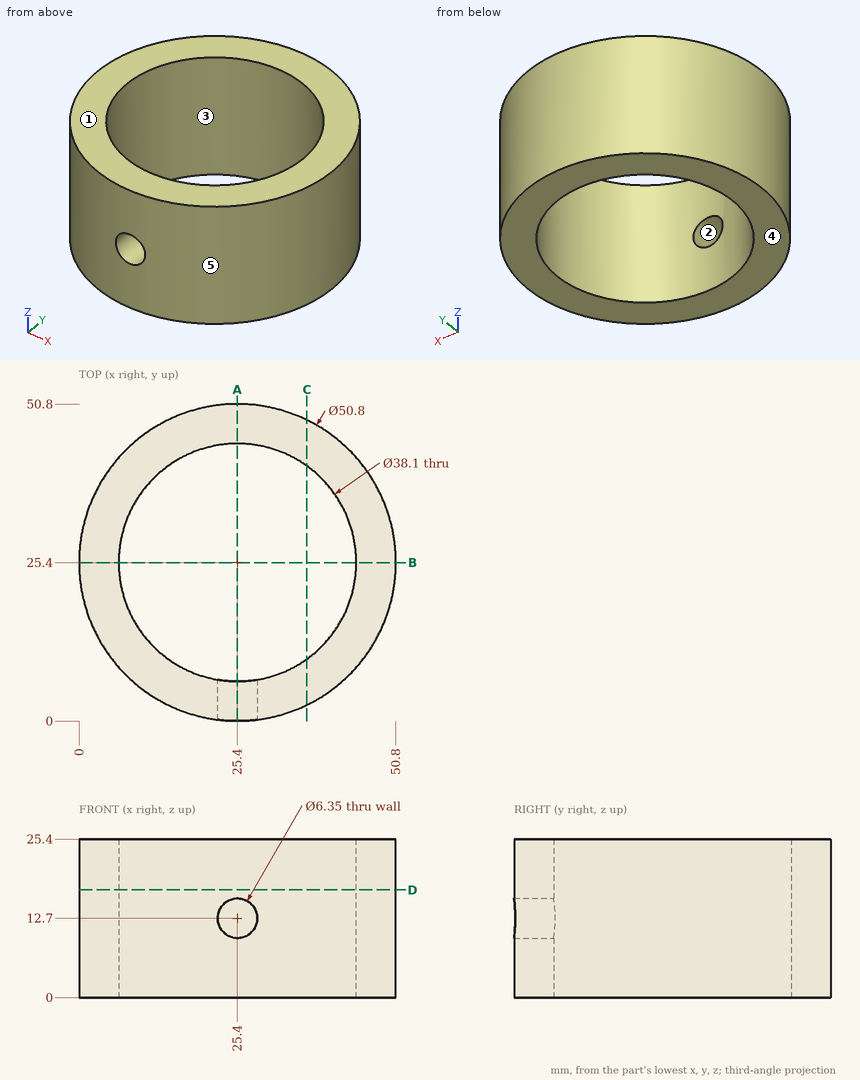
The drawing under review shows one solid part. Ordinate dimensions are in mm from its lowest x, y, z. A direction names the side the tool comes from. Round coordinates to 2 decimals unless told otherwise and drop trailing zeros. Loops run counter-clockwise (first coordinate to the right, second up) from the corner with the lowest first, then second, coordinate; pieces in that order, holes last. Notation, with made-up numbers: (-1.5, 9.5) -> (39.5, 9.5) arc R34 ccw to (39.5, 40.5) -> close; hole circle Ø10 at (-2, 2.25). An arc over 180 degrees is marked (long way). One line per question, with ' | ' between items. Start each with the question number.
Item 1: Add section A-A, the plane x = 25.4. Write out the cut boundary in (y, z) (3 decimals).
Item 2: Draft analysis for pull direction X (two halves, no side actions). For the marked faces 3, 4 and 5, state which applies: +X half, -X half, draft (parallel to the pull), parting line (faces both ways), or undercut.
Item 3: Add section B-B, the plane y = 25.4. Write out the cut boundary in (x, z).
Item 4: Machinability: for the marked faces 1 and 2, which of the approach directions +Z, -Z, +X, -X, +Y, -Y give a long, thin tool a straight path to every point of the face, cutting with its end or side? Answer none if there is none.
Item 5: Wall thickness on line 1 along Y through (x, z) = (25.4, 6); line 2 along Y through (x, z) = (25.4, 11.5); line 3 along X through (y, z) = (35, 10.75): over which ranges is each line inside the solid? List them lowest first. Write a range as [from, to].
Item 6: For pin 1 (4 mm diameter, centred on y = 8.5, z = 11, fed in from +X); pin 2 (1.5 mm diameter, centred on x = 26.5, z = 3, fed in from +Y); pin 3 (1.5 mm diameter, centred on x = 45.5, z = 17, fed in from -Y), all flat-tipped, find the tip position at first contact; note any pin that passes through.
Item 7: Add section C-C, the plane x = 36.5. Write out the cut boundary in (y, z), then the cut area to 3 significant figures.
Item 8: Add section D-D, the plane z = 17.25. Write out the cut boundary in (x, y), then the cut area to 3 significant figures.
Return value:
1) outline: (0, 0) -> (6.35, 0) -> (6.35, 9.525) -> (0, 9.525) -> close; (0, 15.875) -> (6.35, 15.875) -> (6.35, 25.4) -> (0, 25.4) -> close; (44.45, 0) -> (50.8, 0) -> (50.8, 25.4) -> (44.45, 25.4) -> close
2) face 3: undercut | face 4: draft | face 5: parting line
3) outline: (0, 0) -> (6.35, 0) -> (6.35, 25.4) -> (0, 25.4) -> close; (44.45, 0) -> (50.8, 0) -> (50.8, 25.4) -> (44.45, 25.4) -> close
4) face 1: +Z, +X, -X, +Y, -Y | face 2: -Y
5) line 1: y = [0, 6.35], [44.45, 50.8] | line 2: y = [44.45, 50.8] | line 3: x = [1.88, 8.95], [41.85, 48.92]
6) pin 1: stops at x = 45.97 | pin 2: stops at y = 50.8 | pin 3: stops at y = 8.95
7) outline: (2.55, 0) -> (9.92, 0) -> (9.92, 25.4) -> (2.55, 25.4) -> close; (40.88, 0) -> (48.25, 0) -> (48.25, 25.4) -> (40.88, 25.4) -> close | area: 374 mm2
8) outline: circle Ø50.8 at (25.4, 25.4); hole circle Ø38.1 at (25.4, 25.4) | area: 887 mm2
